Drawing for the job (mm, zero at the part's lowest x, y, z). A direction names the side the tool comes from. Round coordinates to 2 decimals unless told otherwise and drop trailing zeros. Write each loop counter-clockwise with the first axis right and the second up, starting at its lowest first coordinate (ties: lowest second). Pieces come first, ordered by that corner, then holes.
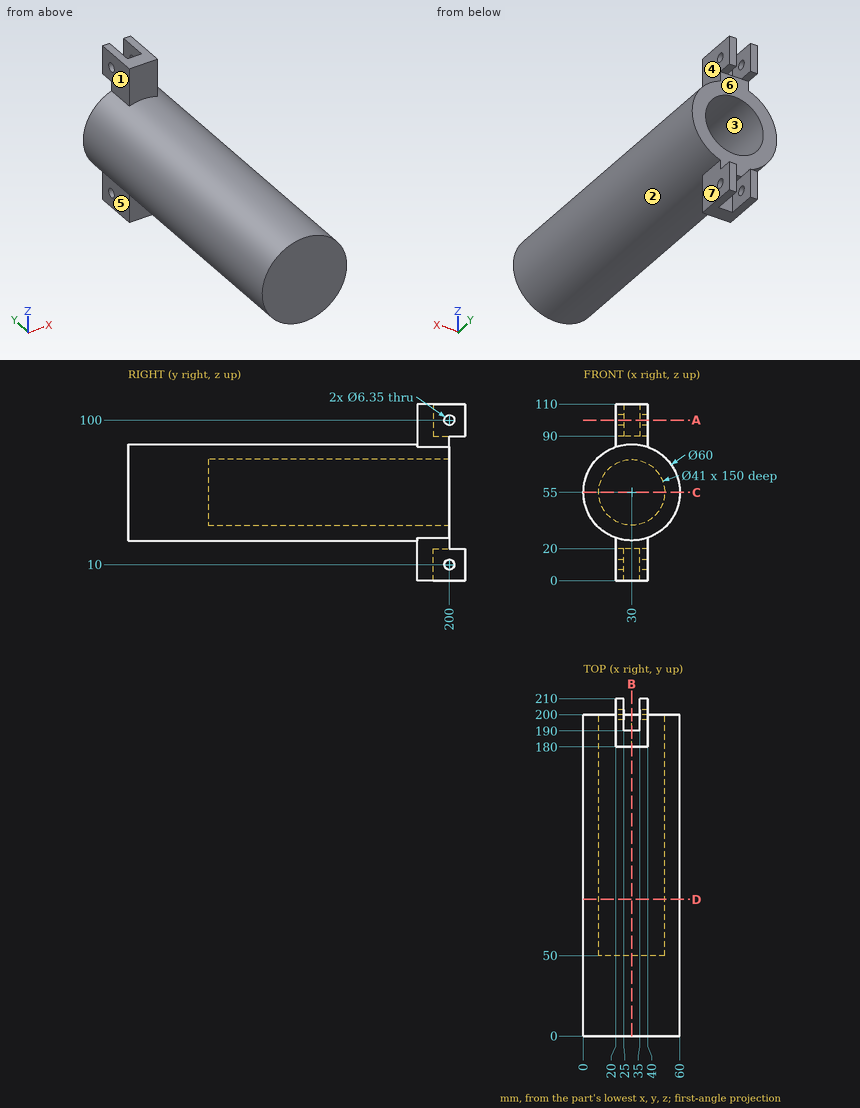
Q1. Saw through at A-A, the plane z = 100. Write the cut outline in (x, y) (3 decimals), and give its area (4 significant figures).
Q2. Drop flat-ended pins along their axis: P1, Ø13.5, axis at y = 200.5, z = 99.5, coming from the +X side; P2, Ø12, axis at x = 12.5, y = 178, coming from the -Z side; P3, Ø1.5, axis at x = 53.5, y = 167, coming from the -Z side; P4, Ø5, axis at y = 200, z = 100, coming from the +X side. Give the stop position or say it passes through.
Q3. Saw through at C-C, the plane z = 55. Write the cut outline in (x, y).
Q4. Saw through at B-B, the plane x = 30. Write the cut outline in (y, z), and give its area (3 significant figures).
Q5. Saw through at D-D, the plane y = 85. Write the cut outline in (x, z), and give its area (3 significant figures).
Q6. Tool access for the marked faces 4, 5, 6 and 7: list every direction of +Z, -Z, +X, -X, +Y, -Y with a clear straight run to the whole face (end or side of a thin tool).
Q7. Two-plate mould, pull along Z, no slides. Class the marked faces 1, 2 and 3: released by +Z, released by -Z, zero draft, split by the parting line, or undercut.
Q8. Wall check: line 1 (Z direction, x = 30, y = 116); line 2 (Y direction, x = 22.05, z = 10) (3 decimals); line 3 (Z direction, x = 36.5, y = 64.5). Give the ranges that are in metal, low to high.
Computed:
1. outline: (20, 180) - (40, 180) - (40, 196.825) - (35, 196.825) - (35, 190) - (25, 190) - (25, 196.825) - (20, 196.825) - close; (20, 203.175) - (25, 203.175) - (25, 210) - (20, 210) - close; (35, 203.175) - (40, 203.175) - (40, 210) - (35, 210) - close
1. area: 336.5 mm2
2. P1: stops at x = 40
2. P2: stops at z = 27.29
2. P3: stops at z = 35.44
2. P4: passes through
3. outline: (0, 0) - (60, 0) - (60, 200) - (50.5, 200) - (50.5, 50) - (9.5, 50) - (9.5, 200) - (0, 200) - close
4. outline: (0, 25) - (180, 25) - (180, 0) - (190, 0) - (190, 20) - (200, 20) - (200, 34.5) - (50, 34.5) - (50, 75.5) - (200, 75.5) - (200, 90) - (190, 90) - (190, 110) - (180, 110) - (180, 85) - (0, 85) - close
4. area: 6,450 mm2
5. outline: circle Ø60 at (30, 55); hole circle Ø41 at (30, 55)
5. area: 1,510 mm2
6. face 4: +Z, +X, +Y, -Y
6. face 5: -Z, -X, +Y, -Y
6. face 6: +X, -X, +Y
6. face 7: -Z, +X, +Y, -Y
7. face 1: zero draft
7. face 2: split by the parting line
7. face 3: undercut
8. line 1: z = 25 to 34.5, 75.5 to 85
8. line 2: y = 180 to 196.825, 203.175 to 210
8. line 3: z = 25.71 to 35.56, 74.44 to 84.29
